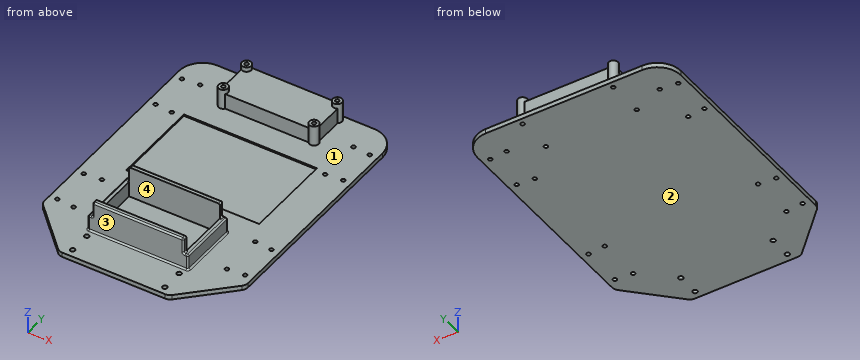
from build123d import *

# Parameters (mm, degrees)
SKETCH_W        = 130
SKETCH_H        = 180
PAD_DEPTH       = 3
CHAMFER_SIZE    = 30
CHAMFER001_SIZE = 30
FILLET_R        = 5
FILLET001_R     = 5
FILLET002_R     = 5
FILLET003_R     = 5
FILLET004_R     = 15
FILLET005_R     = 15
SKETCH003_R     = 3
PAD003_DEPTH    = 13
SKETCH004_R     = 1.25
POCKET002_DEPTH = 16.001
SKETCH005_W     = 85
SKETCH005_H     = 57
POCKET003_DEPTH = 1
SKETCH006_W     = 58
SKETCH006_H     = 3
PAD004_DEPTH    = 20
SKETCH007_W     = 3
SKETCH007_H     = 39
PAD005_DEPTH    = 10
FILLET013_R     = 1
FILLET014_R     = 1
FILLET015_R     = 1
FILLET016_R     = 1
FILLET017_R     = 1
FILLET018_R     = 1
FILLET019_R     = 1
FILLET020_R     = 1
FILLET021_R     = 1
FILLET022_R     = 1
FILLET023_R     = 1
FILLET024_R     = 1
FILLET025_R     = 1
SKETCH008_R     = 1.25
SKETCH008_R_2   = 1
POCKET004_DEPTH = 3.001
SKETCH009_R     = 1.5
POCKET005_DEPTH = 3.001
SKETCH010_W     = 61.6
SKETCH010_H     = 26.6
PAD006_DEPTH    = 10
SKETCH011_R     = 1.25
POCKET006_DEPTH = 16.001
SKETCH012_R     = 1.25
POCKET007_DEPTH = 3.001


with BuildPart() as part:
    # Sketch → Pad (new body)
    with BuildSketch(Plane.XY):
        Rectangle(SKETCH_W, SKETCH_H)
    extrude(amount=PAD_DEPTH)

    # Chamfer
    chamfer_edges = [part.edges().sort_by_distance(p)[0] for p in [
        (65, -90, 1.5),
    ]]
    chamfer(chamfer_edges, length=CHAMFER_SIZE)

    # Chamfer001
    chamfer001_edges = [part.edges().sort_by_distance(p)[0] for p in [
        (-65, -90, 1.5),
    ]]
    chamfer(chamfer001_edges, length=CHAMFER001_SIZE)

    # Fillet
    fillet_edges = [part.edges().sort_by_distance(p)[0] for p in [
        (65, -60, 1.5),
    ]]
    fillet(fillet_edges, radius=FILLET_R)

    # Fillet001
    fillet001_edges = [part.edges().sort_by_distance(p)[0] for p in [
        (35, -90, 1.5),
    ]]
    fillet(fillet001_edges, radius=FILLET001_R)

    # Fillet002
    fillet002_edges = [part.edges().sort_by_distance(p)[0] for p in [
        (-35, -90, 1.5),
    ]]
    fillet(fillet002_edges, radius=FILLET002_R)

    # Fillet003
    fillet003_edges = [part.edges().sort_by_distance(p)[0] for p in [
        (-65, -60, 1.5),
    ]]
    fillet(fillet003_edges, radius=FILLET003_R)

    # Fillet004
    fillet004_edges = [part.edges().sort_by_distance(p)[0] for p in [
        (-65, 90, 1.5),
    ]]
    fillet(fillet004_edges, radius=FILLET004_R)

    # Fillet005
    fillet005_edges = [part.edges().sort_by_distance(p)[0] for p in [
        (65, 90, 1.5),
    ]]
    fillet(fillet005_edges, radius=FILLET005_R)

    # Sketch003 (on Face14 of Fillet005) → Pad003 (join)
    with BuildSketch(Plane.XY.offset(3)):
        with Locations((-29, 86)):
            Circle(SKETCH003_R)
        with Locations((29, 86)):
            Circle(SKETCH003_R)
        with Locations((-29, 63)):
            Circle(SKETCH003_R)
        with Locations((29, 63)):
            Circle(SKETCH003_R)
    extrude(amount=PAD003_DEPTH)

    # Sketch004 (on Face20 of Pad003) → Pocket002 (cut, through all)
    with BuildSketch(Plane.XY.offset(16)):
        with Locations((-29, 86)):
            Circle(SKETCH004_R)
        with Locations((29, 86)):
            Circle(SKETCH004_R)
        with Locations((29, 63)):
            Circle(SKETCH004_R)
        with Locations((-29, 63)):
            Circle(SKETCH004_R)
    extrude(amount=-POCKET002_DEPTH, mode=Mode.SUBTRACT)

    # Sketch005 (on Face18 of Pocket002) → Pocket003 (cut)
    with BuildSketch(Plane.XY.offset(3)):
        with Locations((0, 16.5)):
            Rectangle(SKETCH005_W, SKETCH005_H)
    extrude(amount=-POCKET003_DEPTH, mode=Mode.SUBTRACT)

    # Sketch006 (on Face18 of Pocket003) → Pad004 (join)
    with BuildSketch(Plane.XY.offset(3)):
        with Locations((0, -28.5)):
            Rectangle(SKETCH006_W, SKETCH006_H)
        with Locations((0, -64.5)):
            Rectangle(SKETCH006_W, SKETCH006_H)
    extrude(amount=PAD004_DEPTH)

    # Sketch007 (on Face18 of Pad004) → Pad005 (join)
    with BuildSketch(Plane.XY.offset(3)):
        with Locations((30.5, -46.5)):
            Rectangle(SKETCH007_W, SKETCH007_H)
        with Locations((-30.5, -46.5)):
            Rectangle(SKETCH007_W, SKETCH007_H)
    extrude(amount=PAD005_DEPTH)

    # Fillet013
    fillet013_edges = [part.edges().sort_by_distance(p)[0] for p in [
        (-29, -28.5, 13),
    ]]
    fillet(fillet013_edges, radius=FILLET013_R)

    # Fillet014
    fillet014_edges = [part.edges().sort_by_distance(p)[0] for p in [
        (-29, -64.5, 13),
    ]]
    fillet(fillet014_edges, radius=FILLET014_R)

    # Fillet015
    fillet015_edges = [part.edges().sort_by_distance(p)[0] for p in [
        (-29, -28.5, 23),
    ]]
    fillet(fillet015_edges, radius=FILLET015_R)

    # Fillet016
    fillet016_edges = [part.edges().sort_by_distance(p)[0] for p in [
        (-29, -64.5, 23),
    ]]
    fillet(fillet016_edges, radius=FILLET016_R)

    # Fillet017
    fillet017_edges = [part.edges().sort_by_distance(p)[0] for p in [
        (-32, -46.5, 13),
    ]]
    fillet(fillet017_edges, radius=FILLET017_R)

    # Fillet018
    fillet018_edges = [part.edges().sort_by_distance(p)[0] for p in [
        (-32, -27, 7.5),
    ]]
    fillet(fillet018_edges, radius=FILLET018_R)

    # Fillet019
    fillet019_edges = [part.edges().sort_by_distance(p)[0] for p in [
        (-32, -66, 7.5),
    ]]
    fillet(fillet019_edges, radius=FILLET019_R)

    # Fillet020
    fillet020_edges = [part.edges().sort_by_distance(p)[0] for p in [
        (29, -28.5, 13),
    ]]
    fillet(fillet020_edges, radius=FILLET020_R)

    # Fillet021
    fillet021_edges = [part.edges().sort_by_distance(p)[0] for p in [
        (29, -64.5, 13),
    ]]
    fillet(fillet021_edges, radius=FILLET021_R)

    # Fillet022
    fillet022_edges = [part.edges().sort_by_distance(p)[0] for p in [
        (32, -46.5, 13),
    ]]
    fillet(fillet022_edges, radius=FILLET022_R)

    # Fillet023
    fillet023_edges = [part.edges().sort_by_distance(p)[0] for p in [
        (29, -27, 18),
    ]]
    fillet(fillet023_edges, radius=FILLET023_R)

    # Fillet024
    fillet024_edges = [part.edges().sort_by_distance(p)[0] for p in [
        (29, -66, 18),
    ]]
    fillet(fillet024_edges, radius=FILLET024_R)

    # Fillet025
    fillet025_edges = [part.edges().sort_by_distance(p)[0] for p in [
        (32, -46.5, 3),
    ]]
    fillet(fillet025_edges, radius=FILLET025_R)

    # Sketch008 (on Face10 of Fillet025) → Pocket004 (cut, through all)
    with BuildSketch(Plane.XY.offset(3)):
        with Locations((-60, -52.928932)):
            Circle(SKETCH008_R)
        with Locations((-49, -53.928932)):
            Circle(SKETCH008_R)
        with Locations((-60, -26.928932)):
            Circle(SKETCH008_R)
        with Locations((-49, -25.928932)):
            Circle(SKETCH008_R)
        with Locations((60, -52.928932)):
            Circle(SKETCH008_R)
        with Locations((49, -53.928932)):
            Circle(SKETCH008_R)
        with Locations((60, -26.928932)):
            Circle(SKETCH008_R)
        with Locations((49, -25.928932)):
            Circle(SKETCH008_R)
        with Locations((-60, 70)):
            Circle(SKETCH008_R)
        with Locations((-49, 71)):
            Circle(SKETCH008_R)
        with Locations((-49, 43)):
            Circle(SKETCH008_R)
        with Locations((-60, 44)):
            Circle(SKETCH008_R)
        with Locations((60, 70)):
            Circle(SKETCH008_R_2)
        with Locations((60, 44)):
            Circle(SKETCH008_R_2)
        with Locations((49, 71)):
            Circle(SKETCH008_R)
        with Locations((49, 43)):
            Circle(SKETCH008_R_2)
    extrude(amount=-POCKET004_DEPTH, mode=Mode.SUBTRACT)

    # Sketch009 (on Face10 of Pocket004) → Pocket005 (cut, through all)
    with BuildSketch(Plane.XY.offset(3)):
        with Locations((29.5, -71)):
            Circle(SKETCH009_R)
        with Locations((-29.5, -71)):
            Circle(SKETCH009_R)
        with Locations((-29.5, -85)):
            Circle(SKETCH009_R)
        with Locations((29.5, -85)):
            Circle(SKETCH009_R)
    extrude(amount=-POCKET005_DEPTH, mode=Mode.SUBTRACT)

    # Sketch010 (on Face10 of Pocket005) → Pad006 (join)
    with BuildSketch(Plane.XY.offset(3)):
        with Locations((0, 74.5)):
            Rectangle(SKETCH010_W, SKETCH010_H)
    extrude(amount=PAD006_DEPTH)

    # Sketch011 (on Face86 of Pad006) → Pocket006 (cut, through all)
    with BuildSketch(Plane.XY.offset(16)):
        with Locations((-29, 86)):
            Circle(SKETCH011_R)
        with Locations((29, 86)):
            Circle(SKETCH011_R)
        with Locations((29, 63)):
            Circle(SKETCH011_R)
        with Locations((-29, 63)):
            Circle(SKETCH011_R)
    extrude(amount=-POCKET006_DEPTH, mode=Mode.SUBTRACT)

    # Sketch012 (on Face10 of Pocket006) → Pocket007 (cut, through all)
    with BuildSketch(Plane.XY.offset(3)):
        with Locations((60, 70)):
            Circle(SKETCH012_R)
        with Locations((60, 44)):
            Circle(SKETCH012_R)
        with Locations((49, 43)):
            Circle(SKETCH012_R)
    extrude(amount=-POCKET007_DEPTH, mode=Mode.SUBTRACT)


solid = part.part
Geometry check sheet. Reference: the model listing, model coordinates, mm. Face numbers are marked on the shaded views. A direction names the side the tool comes from. Coordinates: 2 decimals unless noted, no trailing zeros. Order: outer loops, then holes, each group sorted by start corner. A loop starts at its lowest first (then second) coordinate and runs counter-clockwise, first axis right, second up. Notation, with made-up numbers: (78.25, 16) -> (97.25, 16) arc R33 ccw to (97.25, 53) -> close; hole circle Ø11 at (-24, -0.75). An arc over 180 degrees is marked (long way). Use a Markdown table: item, result. Add a question column.
1. Cross-section at B-B (x = -18.5). Enter the section's corners in (y, z), and give its area (3 significant figures).
2. Material ranges on L1, parallel to X at y = -85, z = 1.3; L2, parallel to Y at x = -49, z = 2.25; L3, parallel to X at y = -71, z = 1.2, recorded low to high.
3. Cross-section at A-A (z = 9.5). Enter the section's corners in (x, y), and give its area (3 significant figures).
4. Cross-section at C-C (y = -6). Enter the section's corners in (x, z), and give its area (3 significant figures).
5. Set-up check for the marked faces 1 and 2: record each of +Z, -Z, +X, -X, +Y, -Y from which the full face is reachable in a straight line by a thin tool's end or side.
6. Go/stop test with flat-tipped pins: pin 1 Ø5 at (x, y) = (30, 85.5) entering from +Z; pin 2 Ø3 at (x, y) = (-49, 71) entering from -Z; pin 3 Ø12 at (x, z) = (24, 15.5) entering from -Y; pin 4 Ø4 at (y, z) = (-32, 11) entering from +X. Record where each tip stops, or that it passes through.
7. Cross-section at D-D (x = 39.5). Enter the section's corners in (y, z).
8. Mould release check, pull along X, two halves, no side actions. Record for the marked faces 3 and 4: pulls with the +X half, pulls with the -X half, needs draft (parallel to the pull), parting line crosses it, or undercut.
Filled sheet:
| question | item | result |
|---|---|---|
| 1 | outline | (-90, 0) -> (90, 0) -> (90, 3) -> (87.8, 3) -> (87.8, 13) -> (61.2, 13) -> (61.2, 3) -> (45, 3) -> (45, 2) -> (-12, 2) -> (-12, 3) -> (-26, 3) arc R1 cw to (-27, 4) -> (-27, 22) arc R1 ccw to (-28, 23) -> (-30, 23) -> (-30, 3) -> (-63, 3) -> (-63, 23) -> (-65, 23) arc R1 ccw to (-66, 22) -> (-66, 4) arc R1 cw to (-67, 3) -> (-90, 3) -> close |
| 1 | area | 869 mm2 |
| 2 | L1 | -40 to -31, -28 to 28, 31 to 40 |
| 2 | L2 | -76 to -55.18, -52.68 to -27.18, -24.68 to 41.75, 44.25 to 69.75, 72.25 to 90 |
| 2 | L3 | -54 to -31, -28 to 28, 31 to 54 |
| 3 | outline | (-32, -65) arc R1 ccw to (-31, -66) -> (31, -66) arc R1 ccw to (32, -65) -> (32, -28) arc R1 ccw to (31, -27) -> (-31, -27) arc R1 ccw to (-32, -28) -> close; (-30.8, 65.4) arc R3 ccw (long way) to (-26.6, 61.2) -> (26.6, 61.2) arc R3 ccw (long way) to (30.8, 65.4) -> (30.8, 83.6) arc R3 ccw (long way) to (26.6, 87.8) -> (-26.6, 87.8) arc R3 ccw (long way) to (-30.8, 83.6) -> close; hole circle Ø2.5 at (-29, 63); hole circle Ø2.5 at (-29, 86); hole (-29, -63) -> (29, -63) -> (29, -30) -> (-29, -30) -> close; hole circle Ø2.5 at (29, 63); hole circle Ø2.5 at (29, 86) |
| 3 | area | 2,230 mm2 |
| 4 | outline | (-65, 0) -> (65, 0) -> (65, 3) -> (42.5, 3) -> (42.5, 2) -> (-42.5, 2) -> (-42.5, 3) -> (-65, 3) -> close |
| 4 | area | 305 mm2 |
| 5 | face 1 | +Z |
| 5 | face 2 | -Z, +X, -X, +Y, -Y |
| 6 | pin 1 | z = 16 |
| 6 | pin 2 | z = 0 |
| 6 | pin 3 | y = -66 |
| 6 | pin 4 | x = 32 |
| 7 | outline | (-85.5, 0) -> (90, 0) -> (90, 3) -> (45, 3) -> (45, 2) -> (-12, 2) -> (-12, 3) -> (-85.5, 3) -> close |
| 8 | face 3 | needs draft |
| 8 | face 4 | undercut |
